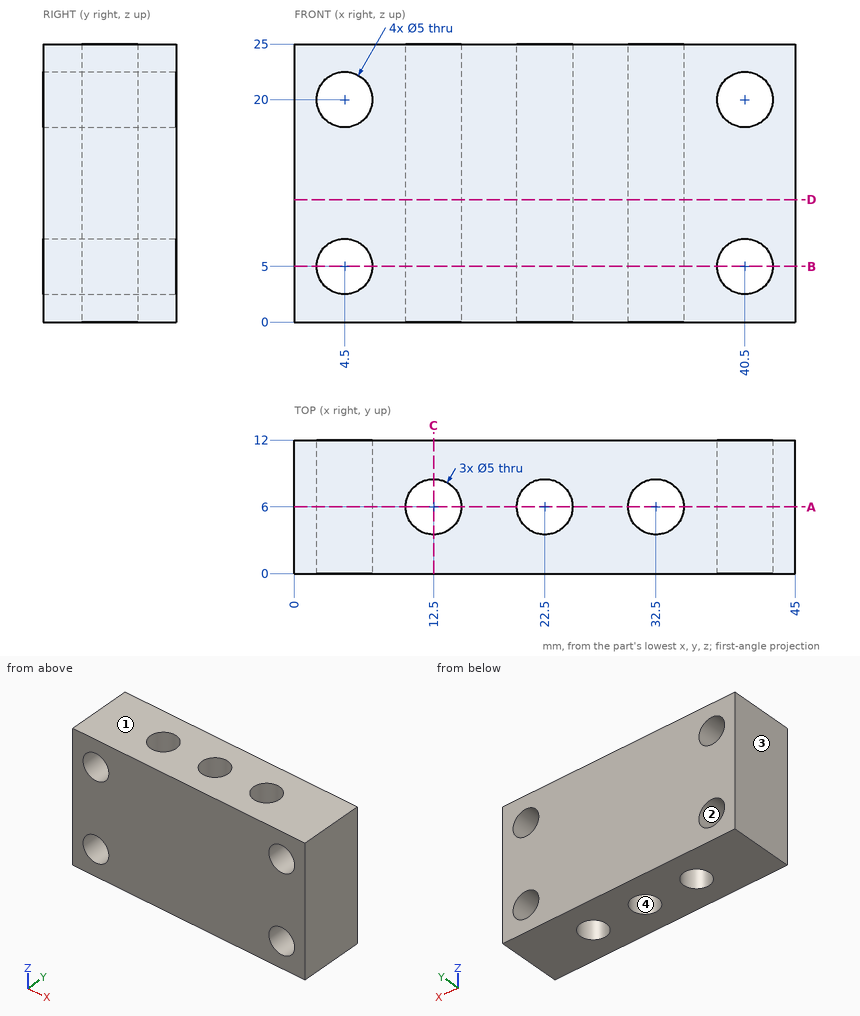
Verification items for this drawing (mm, ordinates from the low corner). Give positions to 0.01 mm unless a question says otherwise; leave off trailing zeros. Loops run counter-clockwise (first coordinate to the right, second up) from the corner with the lowest first, then second, coordinate; pieces in that order, holes last. Notation, with made-up numbers: M -32,12 L -18,12 A22 ccw -18,45 Z; hole C 42,71.25 d7. An arc over 180 degrees is marked long. Write item = value, one per line. Start each with the question number.
1. Section check A-A, the plane y = 6. Enter the section's corners in (x, z).
2. Section check C-C, the plane x = 12.5. Enter the section's corners in (y, z), plus the area to 3 significant figures.
3. Thickness scan on probe 1 along Z at (x, y) = (40.5, 8.5); probe 2 along X at (y, z) = (11.5, 20); probe 3 along X at (y, z) = (6.25, 19). Record the ranges inside material, lowest first.
4. Section check B-B, the plane z = 5. Enter the section's corners in (x, y).
5. Section check D-D, the plane z = 11. Enter the section's corners in (x, y).
6. Draft check along X on the marked faces 1, 2, 3 and 4. Enter one of: +X half, -X half, draft (parallel to the pull), parting line (faces both ways), or undercut.
Values follow:
q1.outline = M 0,0 L 10,0 L 10,25 L 0,25 Z; M 15,0 L 20,0 L 20,25 L 15,25 Z; M 25,0 L 30,0 L 30,25 L 25,25 Z; M 35,0 L 45,0 L 45,25 L 35,25 Z; hole C 4.5,5 d5; hole C 4.5,20 d5; hole C 40.5,5 d5; hole C 40.5,20 d5
q2.outline = M 0,0 L 3.5,0 L 3.5,25 L 0,25 Z; M 8.5,0 L 12,0 L 12,25 L 8.5,25 Z
q2.area = 175 mm^2
q3.probe_1 = 0 to 2.5, 7.5 to 17.5, 22.5 to 25
q3.probe_2 = 0 to 2, 7 to 38, 43 to 45
q3.probe_3 = 0 to 2.21, 6.79 to 10.01, 14.99 to 20.01, 24.99 to 30.01, 34.99 to 38.21, 42.79 to 45
q4.outline = M 0,0 L 2,0 L 2,12 L 0,12 Z; M 7,0 L 38,0 L 38,12 L 7,12 Z; M 43,0 L 45,0 L 45,12 L 43,12 Z; hole C 12.5,6 d5; hole C 22.5,6 d5; hole C 32.5,6 d5
q5.outline = M 0,0 L 45,0 L 45,12 L 0,12 Z; hole C 12.5,6 d5; hole C 22.5,6 d5; hole C 32.5,6 d5
q6.face_1 = draft
q6.face_2 = undercut
q6.face_3 = -X half
q6.face_4 = undercut
